Here's the drawing with two shaded views (mm, measured from the low corner). I have some questions. A direction names the side the tool comes from. Give positions to 0.01 mm unless a question says otherwise; leave off trailing zeros. Order: outer loops, then holes, each group sorted by start corner. A loop starts at its lowest first (then second) coordinate and runs counter-clockwise, first axis right, second up. Notation, with made-up numbers: M 35.5,11.25 L 83.5,11.25 A21 cw 83.5,38.25 Z; hole C -29.5,71.25 d2. An arc over 180 degrees is marked long. Write each question's results on one line, items separated by ' | '.
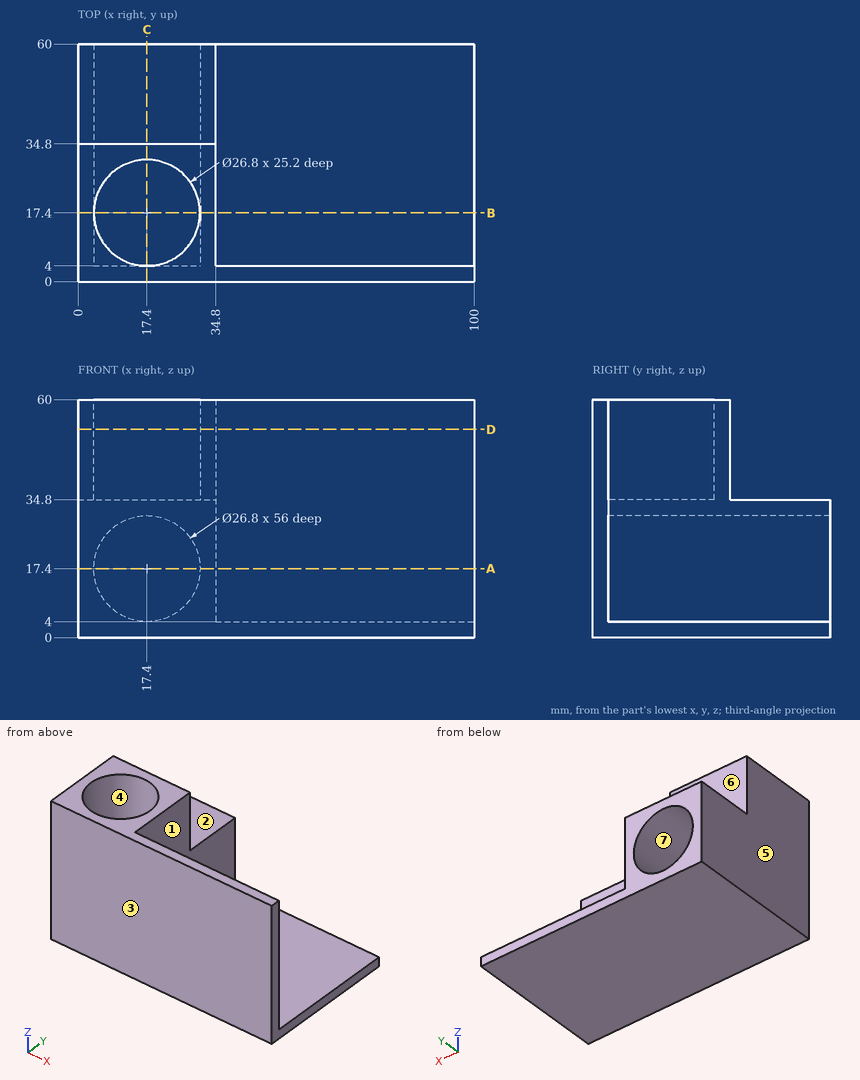
(1) Imagine slicing it at C-C, the plane x = 17.4. Write out the boundary of the cut face in (y, z), plus the area to 3 significant figures.
Data:
outline: M 0,0 L 60,0 L 60,4 L 4,4 L 4,30.8 L 60,30.8 L 60,34.8 L 34.8,34.8 L 34.8,60 L 30.8,60 L 30.8,34.8 L 4,34.8 L 4,60 L 0,60 Z | area: 789 mm2
(2) Will these pins go through, and if not, where does the flat tip stop? P1, Ø10, axis at x = 10, z = 18.5, coming from the +Y side; P2, Ø2, axis at y = 44, z = 15, coming from the +X side; P3, Ø20, axis at x = 16.5, z = 53.5, coming from the +Y side.
Data:
P1: stops at y = 4 | P2: stops at x = 34.8 | P3: stops at y = 34.8
(3) Imagine slicing it at B-B, the plane y = 17.4. Write out the boundary of the cut face in (x, z).
Data:
outline: M 0,0 L 100,0 L 100,4 L 34.8,4 L 34.8,60 L 30.8,60 L 30.8,34.8 L 4,34.8 L 4,60 L 0,60 Z; hole C 17.4,17.4 d26.8
(4) Imagine slicing it at A-A, the plane z = 17.4. Write out the boundary of the cut face in (x, y), plus the area to 3 significant figures.
Data:
outline: M 0,0 L 100,0 L 100,4 L 34.8,4 L 34.8,60 L 30.8,60 L 30.8,4 L 4,4 L 4,60 L 0,60 Z | area: 848 mm2
(5) For the marked faces 1, 2 and 3, which set-ups out of +Z, -Z, +X, -X, +Y, -Y let a thin tool reach every point of the face, with its end or its side?
Data:
face 1: +Z, +X, +Y | face 2: +Z, +X, -X, +Y | face 3: +Z, -Z, +X, -X, -Y
(6) I need wall thicknesses on L1, parallel to X at y = 26, z = 17; L2, parallel to Y at x = 17.4, z = 52; L3, parallel to Z at x = 89, y = 56.5. Which ranges of each line are inside material? Lowest first, please. Write a range as from..to.
Data:
L1: x = 0..4.01, 30.79..34.8 | L2: y = 0..4, 30.8..34.8 | L3: z = 0..4
(7) We'd pull the mould along X, two halves only. Please class the marked faces 4, 5, 6 and 7: +X half, -X half, draft (parallel to the pull), parting line (faces both ways), or undercut.
Data:
face 4: undercut | face 5: -X half | face 6: draft | face 7: undercut
(8) Imagine slicing it at D-D, the plane z = 52.5. Write out the boundary of the cut face in (x, y).
Data:
outline: M 0,0 L 100,0 L 100,4 L 34.8,4 L 34.8,34.8 L 0,34.8 Z; hole C 17.4,17.4 d26.8
